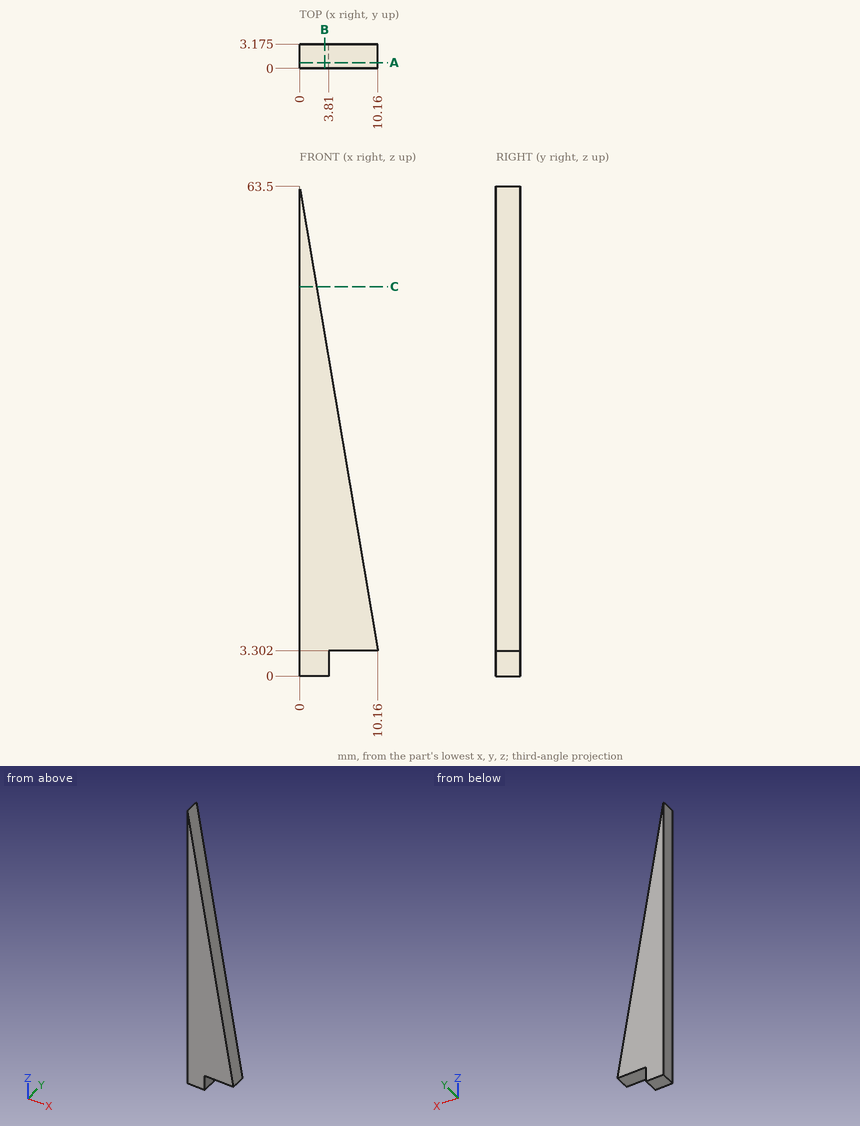
Check sheet for the drawn part. Datum: minimum x, y, z corner. Units: mm. Coordinates: 2 decimals unless noted, no trailing zeros. Loops run counter-clockwise (first coordinate to the right, second up) from the corner with the lowest first, then second, coordinate; pieces in that order, holes last. Notation, with made-up numbers: (-36.5, 26) -> (-2.5, 26) arc R9 cw to (-2.5, 40) -> close; hole circle Ø7 at (79.25, 33.25). An arc over 180 degrees is marked (long way). Answer in a Markdown table with one row per item.
1) Section check B-B (x = 3.25). Record the cut outline in (y, z) (3 decimals), and give its area (3 significant figures).
The answers:
| item | result |
|---|---|
| outline | (0, 0) -> (3.175, 0) -> (3.175, 44.244) -> (0, 44.244) -> close |
| area | 140 mm2 |
2) Section check A-A (y = 0.75). Record the cut outline in (x, z).
The answers:
| item | result |
|---|---|
| outline | (0, 0) -> (3.81, 0) -> (3.81, 3.3) -> (10.16, 3.3) -> (0, 63.5) -> close |
3) Scan lines: line 1 along X through (y, z) = (0.65, 43); line 2 along X through (y, z) = (1.15, 49). Record each from-to range of solid material in increasing order. Write a range as from..to.
The answers:
| item | result |
|---|---|
| line 1 | x = 0..3.46 |
| line 2 | x = 0..2.45 |
4) Section check C-C (z = 50.5). Record the cut outline in (x, y) (3 decimals).
The answers:
| item | result |
|---|---|
| outline | (0, 0) -> (2.194, 0) -> (2.194, 3.175) -> (0, 3.175) -> close |
5) Depth check by flat-ended pin: P1, Ø1.6, axis at x = 8, y = 1, coming from the -Z side. Enter the tip coordinate at first touch or a pass-through.
The answers:
| item | result |
|---|---|
| P1 | stops at z = 3.3 |
